from build123d import *

# Parameters (mm, degrees)
SKETCH1_R           = 0.425
SKETCH1_R_2         = 0.8
BOSS_EXTRUDE1_DEPTH = 1.6
CUT_EXTRUDE1_DEPTH  = 0.0001
CUT_EXTRUDE2_DEPTH  = 0.0001
PARTFOOTPRINTS_W    = 30.48
PARTFOOTPRINTS_H    = 7.989227112
PARTFOOTPRINTS_W_2  = 3.5
PARTFOOTPRINTS_H_2  = 6.95
CUT_EXTRUDE3_DEPTH  = 0.0001
CUT_EXTRUDE4_DEPTH  = 71.235674696
SKETCH3_W           = 7.779754111
SKETCH3_H           = 5.155241991
CUT_EXTRUDE5_DEPTH  = 10
FILLET1_R           = 1


with BuildPart() as part:
    # Sketch1 → Boss-Extrude1 (new body)
    with BuildSketch(Plane(origin=(0, 0, -0.0125), x_dir=(-1, 0, 0), z_dir=(0, 0, -1))):
        with BuildLine():
            Line((35.3, -50), (35.3, -48))
            ThreePointArc((35.3, -48), (35.592893219, -47.292893219), (36.3, -47))
            Line((36.3, -47), (45.8, -47))
            ThreePointArc((45.8, -47), (46.507106781, -46.707106781), (46.8, -46))
            Line((46.8, -46), (46.8, -41.4))
            ThreePointArc((46.8, -41.4), (47.092893219, -40.692893219), (47.8, -40.4))
            Line((47.8, -40.4), (49.3, -40.4))
            Line((49.3, -40.4), (49.3, 39.2))
            Line((49.3, 39.2), (43.2, 45.3))
            Line((43.2, 45.3), (35.500000002, 45.3))
            Line((35.500000002, 45.3), (35.500000002, 43.8))
            ThreePointArc((35.500000002, 43.8), (35.207106783, 43.092893219), (34.500000002, 42.8))
            Line((34.500000002, 42.8), (4.499999998, 42.8))
            ThreePointArc((4.499999998, 42.8), (3.792893217, 43.092893219), (3.499999998, 43.8))
            Line((3.499999998, 43.8), (3.499999998, 45.3))
            Line((3.499999998, 45.3), (-43.2, 45.3))
            Line((-43.2, 45.3), (-49.3, 39.2))
            Line((-49.3, 39.2), (-49.3, -40.4))
            Line((-49.3, -40.4), (-47.8, -40.4))
            ThreePointArc((-47.8, -40.4), (-47.092893219, -40.692893219), (-46.8, -41.4))
            Line((-46.8, -41.4), (-46.8, -46))
            ThreePointArc((-46.8, -46), (-46.507106781, -46.707106781), (-45.8, -47))
            Line((-45.8, -47), (-36.3, -47))
            ThreePointArc((-36.3, -47), (-35.592893219, -47.292893219), (-35.3, -48))
            Line((-35.3, -48), (-35.3, -50))
            Line((-35.3, -50), (35.3, -50))
        make_face()
        with Locations(Location((-21.27, 41.37, 0), (0, 0, 180))):
            Circle(SKETCH1_R, mode=Mode.SUBTRACT)
        with Locations(Location((-23.81, 41.37, 0), (0, 0, 180))):
            Circle(SKETCH1_R, mode=Mode.SUBTRACT)
        with Locations(Location((-22.54, 40.1, 0), (0, 0, 180))):
            Circle(SKETCH1_R, mode=Mode.SUBTRACT)
        with Locations(Location((-13.87, 41.37, 0), (0, 0, 180))):
            Circle(SKETCH1_R, mode=Mode.SUBTRACT)
        with Locations(Location((-23.81, 38.83, 0), (0, 0, 180))):
            Circle(SKETCH1_R, mode=Mode.SUBTRACT)
        with Locations(Location((-16.41, 41.37, 0), (0, 0, 180))):
            Circle(SKETCH1_R, mode=Mode.SUBTRACT)
        with Locations(Location((-15.14, 40.1, 0), (0, 0, 180))):
            Circle(SKETCH1_R, mode=Mode.SUBTRACT)
        with Locations(Location((-21.27, 38.83, 0), (0, 0, 180))):
            Circle(SKETCH1_R, mode=Mode.SUBTRACT)
        with Locations(Location((-28.67, 41.37, 0), (0, 0, 180))):
            Circle(SKETCH1_R, mode=Mode.SUBTRACT)
        with Locations(Location((-31.21, 41.37, 0), (0, 0, 180))):
            Circle(SKETCH1_R, mode=Mode.SUBTRACT)
        with Locations(Location((-16.41, 38.83, 0), (0, 0, 180))):
            Circle(SKETCH1_R, mode=Mode.SUBTRACT)
        with Locations(Location((-29.94, 40.1, 0), (0, 0, 180))):
            Circle(SKETCH1_R, mode=Mode.SUBTRACT)
        with Locations(Location((-31.21, 38.83, 0), (0, 0, 180))):
            Circle(SKETCH1_R, mode=Mode.SUBTRACT)
        with Locations(Location((-28.67, 38.83, 0), (0, 0, 180))):
            Circle(SKETCH1_R, mode=Mode.SUBTRACT)
        with Locations(Location((33.775, 38.54, 0), (0, 0, 180))):
            Circle(SKETCH1_R_2, mode=Mode.SUBTRACT)
        with Locations((5.225, 38.54)):
            Circle(SKETCH1_R_2, mode=Mode.SUBTRACT)
        with Locations(Location((-13.87, 38.83, 0), (0, 0, 180))):
            Circle(SKETCH1_R, mode=Mode.SUBTRACT)
    extrude(amount=-BOSS_EXTRUDE1_DEPTH)

    # thermalContacts_lower → Cut-Extrude1 (cut)
    with BuildSketch(Plane(origin=(0, 0, -0.0125), x_dir=(-1, 0, 0), z_dir=(0, 0, -1))):
        Polygon((47, 35.5), (47, -41.5), (59.827263463, -41.5), (59.827263463, 47), (41.5, 47), (41.5, 41.5), (41.5, 35.5), align=None)
        Polygon((-47, 35.5), (-47, -41.5), (-56.192158269, -41.5), (-56.192158269, 47), (-41.5, 47), (-41.5, 41.5), (-41.5, 35.5), align=None)
    extrude(amount=-CUT_EXTRUDE1_DEPTH, mode=Mode.SUBTRACT)

    # thermalContacts_upper → Cut-Extrude2 (cut)
    with BuildSketch(Plane.XY.offset(1.5875)):
        Polygon((-47, 35.5), (-47, -41.5), (-56.192158269, -41.5), (-56.192158269, 47), (-41.5, 47), (-41.5, 41.5), (-41.5, 35.5), align=None)
        Polygon((47, 35.5), (47, -41.5), (59.827263463, -41.5), (59.827263463, 47), (41.5, 47), (41.5, 41.5), (41.5, 35.5), align=None)
    extrude(amount=-CUT_EXTRUDE2_DEPTH, mode=Mode.SUBTRACT)

    # partFootprints → Cut-Extrude3 (cut)
    with BuildSketch(Plane.XY.offset(1.5875)):
        with Locations((-19.5, 38.834613556)):
            Rectangle(PARTFOOTPRINTS_W, PARTFOOTPRINTS_H)
        with Locations((15.14, 41.825)):
            Rectangle(PARTFOOTPRINTS_W_2, PARTFOOTPRINTS_H_2)
        with Locations((22.54, 41.825)):
            Rectangle(PARTFOOTPRINTS_W_2, PARTFOOTPRINTS_H_2)
        with Locations((29.94, 41.825)):
            Rectangle(PARTFOOTPRINTS_W_2, PARTFOOTPRINTS_H_2)
    extrude(amount=-CUT_EXTRUDE3_DEPTH, mode=Mode.SUBTRACT)

    # Sketch2 → Cut-Extrude4 (cut, through all)
    with BuildSketch(Plane.XY.offset(1.5875)):
        with BuildLine():
            Line((29.2, -42.8), (29.2, -40.414213562))
            ThreePointArc((29.2, -40.414213562), (29.2, -39), (30.614213562, -39))
            Line((30.614213562, -39), (31.485786438, -39))
            ThreePointArc((31.485786438, -39), (32.9, -39), (32.9, -40.414213562))
            Line((32.9, -40.414213562), (32.9, -42.8))
            Line((32.9, -42.8), (36.05, -42.8))
            Line((36.05, -42.8), (36.05, -50))
            Line((36.05, -50), (26.05, -50))
            Line((26.05, -50), (26.05, -42.8))
            Line((26.05, -42.8), (29.2, -42.8))
        make_face()
    extrude(amount=-CUT_EXTRUDE4_DEPTH, mode=Mode.SUBTRACT)

    # Sketch3 → Cut-Extrude5 (cut)
    with BuildSketch(Plane.XY.offset(1.5875)):
        with Locations((35.630924609, -49.577620995)):
            Rectangle(SKETCH3_W, SKETCH3_H)
    extrude(amount=-CUT_EXTRUDE5_DEPTH, mode=Mode.SUBTRACT)

    # Fillet1
    fillet1_edges = [part.edges().sort_by_distance(p)[0] for p in [
        (26.05, -50, 0.7875),
        (26.05, -42.8, 0.7875),
        (36.05, -42.8, 0.7875),
        (36.05, -47, 0.7875),
    ]]
    fillet(fillet1_edges, radius=FILLET1_R)


solid = part.part
The model under review builds one solid part; all positions refer to its coordinate system, in mm. Round coordinates to 2 decimals unless told otherwise and drop trailing zeros. Order: outer loops, then holes, each group sorted by start corner. A loop starts at its lowest first (then second) coordinate and runs counter-clockwise, first axis right, second up. Notation, with made-up numbers: (23.5, 3) -> (74.5, 3) arc R28 cw to (74.5, 25) -> close; hole circle Ø7 at (58, -8.5). An arc over 180 degrees is marked (long way). Return JSON: item names as keys, results as strings.
1. Insertion check: P1, Ø0.8, axis at y = -45, z = 0.5, coming from the -X side. The pin has a flat end and moves straight along its axis. Give the tip position at first contact, or say it passes through.
Answer block:
{"P1": "stops at x = -46.8"}
2. Take a section at C-C (x = 39). Write out the cut boundary in (y, z), then the cut area to 3 significant figures.
Answer block:
{"outline": "(-47, -0.01) -> (45.3, -0.01) -> (45.3, 1.59) -> (-47, 1.59) -> close", "area": "148 mm²"}
3. For L1, parallel to Y at x = 28.67, z = 0.7 (3 decimals); L2, parallel to Y at x = 16.41, z = 0.85 (3 decimals); L3, parallel to X at y = -44, z = 0.4, list the stretches that pass through material, from the lowest coordinate up. Write a range as [from, to].
Answer block:
{"L1": "y = [-42.8, 38.405], [39.255, 40.945], [41.795, 45.3]", "L2": "y = [-50, 38.405], [39.255, 40.945], [41.795, 45.3]", "L3": "x = [-46.8, 26.05], [36.05, 46.8]"}
4. Take a section at A-A (z = 0.5). State how many separate pieces and enclosed holes the cut face has, then the cut area to 3 significant figures.
Answer block:
{"separate pieces": "1", "enclosed holes": "17", "area": "9,070 mm²"}
